Here's the drawing with two shaded views (mm, measured from the low corner). I have some questions. Coordinates: 2 decimals unless noted, no trailing zeros. Write each loop counter-clockwise with the first axis right and the second up, starting at its lowest first coordinate (ties: lowest second). Pieces come first, ordered by that corner, then holes.
Item 1: If I drill on line 1 (X direction, y = 4.05, z = 0.15) (3 decimals); line 2 (Y direction, x = 3, z = 0.3); line 3 (Z direction, x = 5.5, y = 3.7), over which ranges is the centre line in solid material (lowest first)?
Item 2: If we section it at A-A (z = 0.55): Please give me the cut outline in (x, y) (3 decimals).
Item 3: I'm going to push a flat-ended pin straight in: pin 1 Ø0.5 at (x, z) = (10.5, 0.5) entering from +Y. Where does the tip first touch, or does it pass through?
Item 4: If we section it at C-C (x = 3.5): Please give me the cut outline in (y, z).
Item 5: If we section it at B-B (y = 4.15): Please give me the cut outline in (x, z) (3 decimals).
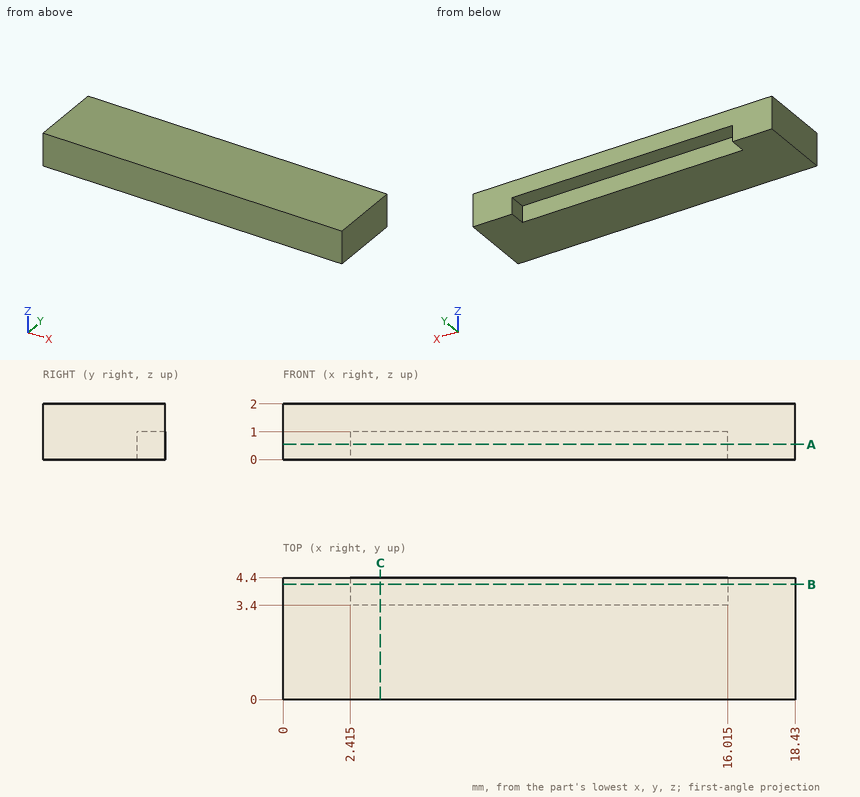
Answer list:
1. line 1: x = 0 to 2.415, 16.015 to 18.43
1. line 2: y = 0 to 3.4
1. line 3: z = 1 to 2
2. outline: (0, 0) - (18.43, 0) - (18.43, 4.4) - (16.015, 4.4) - (16.015, 3.4) - (2.415, 3.4) - (2.415, 4.4) - (0, 4.4) - close
3. pin 1: stops at y = 3.4
4. outline: (0, 0) - (3.4, 0) - (3.4, 1) - (4.4, 1) - (4.4, 2) - (0, 2) - close
5. outline: (0, 0) - (2.415, 0) - (2.415, 1) - (16.015, 1) - (16.015, 0) - (18.43, 0) - (18.43, 2) - (0, 2) - close
